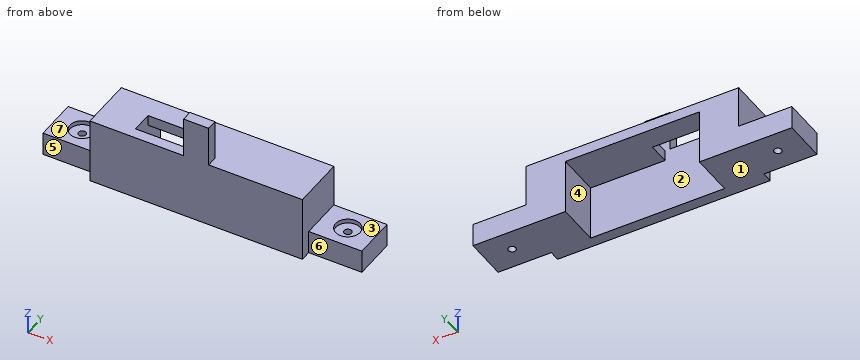
Autodesk Inventor part; units mm, degrees
ref_plane "YZ Plane" through (0, 0, 0) normal (1, 0, 0) x (0, 1, 0)
ref_plane "XZ Plane" through (0, 0, 0) normal (0, 1, 0) x (-1, 0, 0)
ref_plane "XY Plane" through (0, 0, 0) normal (0, 0, 1) x (1, 0, 0)
sketch "Sketch1" plane through (0, 0, 0) normal (0, 1, 0) x (-1, 0, 0)
  line L0 (50, -15.5) -> (-50, -15.5)
  line L1 (-50, -15.5) -> (-50, 15.5)
  line L2 (-50, 15.5) -> (50, 15.5)
  line L3 (50, 15.5) -> (50, -15.5)
  line L4 (31.5, -15.5) -> (-31.5, -15.5)
  line L5 (-31.5, -15.5) -> (-31.5, 10.5)
  line L6 (-31.5, 10.5) -> (31.5, 10.5)
  line L7 (31.5, 10.5) -> (31.5, -15.5)
  line L8 (50, -15.5) -> (75, -15.5)
  line L9 (75, -15.5) -> (75, -4.5)
  line L10 (75, -4.5) -> (50, -4.5)
  line L11 (50, -4.5) -> (50, -15.5)
  line L12 (0, 0) -> (0, -15.5)
  line L13 (-50, -15.5) -> (-75, -15.5)
  line L14 (-75, -15.5) -> (-75, -4.5)
  line L15 (-75, -4.5) -> (-50, -4.5)
  point P0 (-50, -4.5)
  point P1 (-31.5, -15.5)
  dimension "d0" = 100
  dimension "d1" = 50
  dimension "d2" = 31
  dimension "d3" = 15.5
  dimension "d4" = 26
  dimension "d5" = 63
  dimension "d6" = 31.5
  dimension "d7" = 11
  dimension "d8" = 25
extrude "Extrusion1" add sketch "Sketch1" along normal blind 20 contours L0 L7 L6 L5 L1 L2 L3 | L3 L10 L9 L8 | L13 L14 L15 L1
sketch "Sketch2" plane through (-75, 0, -4.5) normal (0, 0, 1) x (1, 0, 0)
  line L0 (0, 0) -> (25, 0)
  line L1 (25, 0) -> (25, 20)
  line L2 (0, 20) -> (25, 20)
  line L3 (0, 0) -> (0, 20)
  circle A0 centre (12.5, 10) radius 1.75
  circle A1 centre (12.5, 10) radius 5.75
  point P0 (75, 0)
  dimension "d11" = 3.5
  dimension "d12" = 11.5
extrude "Extrusion2" cut sketch "Sketch2" against normal through all contours A0
extrude "Extrusion3" cut sketch "Sketch2" against normal blind 2 contours A1
mirror "Mirror1" about plane through (0, 0, 0) normal (1, 0, 0) of "Extrusion3", "Extrusion2"
sketch "Sketch4" plane through (0, 0, 0) normal (0, -1, 0) x (1, 0, 0)
  line L0 (-31.5, -15.5) -> (-75, -15.5)
  line L1 (-31.5, 10.5) -> (-31.5, -15.5)
  line L2 (31.5, 10.5) -> (-31.5, 10.5)
  line L3 (31.5, -15.5) -> (31.5, 10.5)
  line L4 (75, -15.5) -> (31.5, -15.5)
  line L5 (75, -4.5) -> (75, -15.5)
  line L6 (50, -4.5) -> (75, -4.5)
  line L7 (50, 15.5) -> (50, -4.5)
  line L8 (-50, 15.5) -> (50, 15.5)
  line L9 (-50, -4.5) -> (-50, 15.5)
  line L10 (-75, -4.5) -> (-50, -4.5)
  line L11 (-75, -15.5) -> (-75, -4.5)
  line L12 (75, -15.5) -> (31.5, -15.5)
  line L13 (50, -15.5) -> (-50, -15.5)
  line L14 (-50, -15.5) -> (-50, 34.5)
  line L15 (-50, 34.5) -> (50, 34.5)
  line L16 (50, 34.5) -> (50, -15.5)
  point P0 (0, 0)
  dimension "d22" = 100
  dimension "d23" = 50
extrude "Extrusion5" add sketch "Sketch4" along normal blind 5 contours L0 L14 L9 L8 L7 L16 L4 L3 L2 L1 | L1 L2 L3 L13 | L14 L15 L16 L8
sketch "Sketch5" plane through (31.5, 20, 10.5) normal (0, 0, -1) x (-1, 0, 0)
  line L0 (63, -20) -> (0, -20)
  line L1 (63, -20) -> (35, -20)
  line L2 (35, -20) -> (35, -10)
  line L3 (35, -10) -> (63, -10)
  line L4 (63, -10) -> (63, -20)
  point P0 (31.5, -20)
  dimension "d26" = 28
  dimension "d27" = 10
extrude "Extrusion6" cut sketch "Sketch5" against normal blind 57
sketch "Sketch6" plane through (0, 0, 0) normal (0, 1, 0) x (1, 0, 0)
  line L0 (-50, -15.5) -> (-31.5, -15.5)
  line L1 (-50, -34.5) -> (-50, -15.5)
  line L2 (50, -34.5) -> (-50, -34.5)
  line L3 (50, -15.5) -> (50, -34.5)
  line L4 (-3.5, -15.5) -> (50, -15.5)
  line L5 (-3.5, -10.5) -> (-3.5, -15.5)
  line L6 (31.5, -10.5) -> (-3.5, -10.5)
  line L7 (31.5, 15.5) -> (31.5, -10.5)
  line L8 (-31.5, 15.5) -> (31.5, 15.5)
  line L9 (-31.5, 15.5) -> (-31.5, -15.5)
  line L10 (-0.0641, -15.5) -> (-0.0641, -32.5)
  line L11 (-0.0641, -32.5) -> (-0.0641, -22.5) construction
  line L12 (0.7628, -32.5) -> (0.7628, -22.5)
  line L13 (-0.891, -22.5) -> (-0.891, -32.5)
  arc A0 (-0.891, -32.5) -> (0.7628, -32.5) centre (-0.0641, -32.5) ccw
  arc A1 (0.7628, -22.5) -> (-0.891, -22.5) centre (-0.0641, -22.5) ccw
  point P0 (0, 0)
  point P1 (-0.0641, -27.5)
  dimension "d36" = 10
  dimension "d37" = 2
extrude "Extrusion7" cut sketch "Sketch6" against normal blind 2 contours A1 L12 A0 L13
sketch "Sketch7" plane through (0, 0, 0) normal (0, 1, 0) x (1, 0, 0)
  line L0 (-3.5, -10.5) -> (-3.5, -15.5)
  arc A0 (-0.891, -32.5) -> (0.7628, -32.5) centre (-0.0641, -32.5) ccw
  line L1 (-0.891, -32.5) -> (-0.891, -22.5)
  arc A1 (0.7628, -22.5) -> (-0.891, -22.5) centre (-0.0641, -22.5) ccw
  line L2 (0.7628, -22.5) -> (0.7628, -32.5)
  line L3 (-50, -15.5) -> (-31.5, -15.5)
  line L4 (-50, -34.5) -> (-50, -15.5)
  line L5 (50, -34.5) -> (-50, -34.5)
  line L6 (50, -15.5) -> (50, -34.5)
  line L7 (-3.5, -15.5) -> (50, -15.5)
  line L8 (-3.5, -10.5) -> (-3.5, -15.5)
  line L9 (31.5, -10.5) -> (-3.5, -10.5)
  line L10 (31.5, 15.5) -> (31.5, -10.5)
  line L11 (-31.5, 15.5) -> (31.5, 15.5)
  line L12 (-31.5, 15.5) -> (-31.5, -15.5)
  line L13 (-3.5, -15.5) -> (50, -15.5)
  line L14 (50, -34.5) -> (-50, -34.5)
  line L15 (-3.5, -15.5) -> (-50, -15.5)
  line L16 (-50, -15.5) -> (-50, -34.5)
  line L17 (-50, -34.5) -> (-3.5, -34.5)
  line L18 (-3.5, -34.5) -> (-3.5, -15.5)
  line L19 (-50, -15.5) -> (50, -15.5)
  line L20 (-5.891, -34.5) -> (-50, -34.5)
  line L21 (-50, -34.5) -> (-50, -15.5)
  line L22 (-50, -15.5) -> (-5.891, -15.5)
  line L23 (-5.891, -15.5) -> (-5.891, -34.5)
  point P0 (0, 0)
  point P1 (-5.891, -34.5)
  point P2 (-5.891, -15.5)
  dimension "d32" = 5
extrude "Extrusion8" cut sketch "Sketch7" against normal blind 24.25 contours L23 L5 L4 L3 L15
mirror "Mirror2" about plane through (0, 0, 0) normal (1, 0, 0) of "Extrusion8"
sketch "Sketch10" plane through (0, 0, 0) normal (0, 1, 0) x (1, 0, 0)
  line L0 (-3.5, -10.5) -> (-3.5, -15.5)
  arc A0 (0.7628, -22.5) -> (-0.891, -22.5) centre (-0.0641, -22.5) ccw
  line L1 (0.7628, -22.5) -> (0.7628, -32.5)
  arc A1 (-0.891, -32.5) -> (0.7628, -32.5) centre (-0.0641, -32.5) ccw
  line L2 (-0.891, -32.5) -> (-0.891, -22.5)
  line L3 (5.891, -34.5) -> (5.891, -15.5)
  line L4 (-3.5, -15.5) -> (5.891, -15.5)
  line L5 (-3.5, -10.5) -> (-3.5, -15.5)
  line L6 (31.5, -10.5) -> (-3.5, -10.5)
  line L7 (31.5, 15.5) -> (31.5, -10.5)
  line L8 (-31.5, 15.5) -> (31.5, 15.5)
  line L9 (-31.5, 15.5) -> (-31.5, -15.5)
  line L10 (-31.5, -15.5) -> (-5.891, -15.5)
  line L11 (-5.891, -15.5) -> (-5.891, -34.5)
  line L12 (5.891, -34.5) -> (-5.891, -34.5)
  line L13 (-3.5, -15.5) -> (3.4148, -15.5)
  line L14 (3.4148, -15.5) -> (3.4148, -19.7081)
  line L15 (3.4148, -19.7081) -> (-3.5, -19.7081)
  line L16 (-3.5, -19.7081) -> (-3.5, -15.5)
  point P0 (0, 0)
equation "\"d1\" = 0.5 * d0"
equation "\"d3\" = 0.5 * d2"
equation "\"d6\" = 0.5 * d5"
properties part number "blah"
Work out the finished part from the listing and answer in its coordinate system (mm). Face numbers are marked on the shaded views. A direction names the side the tool comes from. Give positions to 0.01 mm unless a question says otherwise; leave off trailing zeros. Loops run counter-clockwise (first coordinate to the right, second up) from the corner with the lowest first, then second, coordinate; pieces in that order, holes last. Notation, with made-up numbers: (13, 64.25) - (30, 64.25) arc R22 ccw to (30, 81.25) - close; hole circle Ø1 at (-23, 17). An arc over 180 degrees is marked (long way). Answer in a Markdown table with one row per item.
(1) A tool of negligible diameter and unlimited length cuts with its end or side. For the marked faces 3, 4, 5, 6 and 7, from which of +Z, -Z, +X, -X, +Y, -Y can it reach the whole face along a straight path? Write none if from no direction.
Results list:
| item | result |
|---|---|
| face 3 | +Z, +X, +Y, -Y |
| face 4 | -Z, +Y |
| face 5 | +Z, -Z, -X, -Y |
| face 6 | +Z, -Z, +X, -Y |
| face 7 | +Z, -X, +Y, -Y |
(2) Section C-C (z = -10) is taken. Give the vertices of the cut face in (x, y), and give its area (3 significant figures).
Results list:
| item | result |
|---|---|
| outline | (-75, 0) - (-50, 0) - (-50, -5) - (50, -5) - (50, 0) - (75, 0) - (75, 20) - (31.5, 20) - (31.5, 0) - (-31.5, 0) - (-31.5, 20) - (-75, 20) - close; hole circle Ø3.5 at (-62.5, 10); hole circle Ø3.5 at (62.5, 10) |
| area | 2,220 mm² |
(3) Consider L1, parallel to X at y = 9.5, z = -5.5; L2, parallel to X at y = 6.25, z = 14.5; L3, parallel to X at y = 7.75, z = 10. Determine where each line is inside the solid, lowest interval first. Write a range as [from, to].
Results list:
| item | result |
|---|---|
| L1 | x = [-75, -68.23], [-56.77, -31.5], [31.5, 56.77], [68.23, 75] |
| L2 | x = [-50, -31.5], [-3.5, 50] |
| L3 | x = [-50, -31.5], [31.5, 50] |
(4) Section D-D (z = -1) is taken. Give the vertices of the cut face in (x, y).
Results list:
| item | result |
|---|---|
| outline | (-50, -5) - (50, -5) - (50, 20) - (31.5, 20) - (31.5, 0) - (-31.5, 0) - (-31.5, 20) - (-50, 20) - close |
(5) For a pull along X with two mould halves and no side action, classify the marked faces 1 and 2 as pulls with the +X half, pulls with the -X half, needs draft (parallel to the pull), parting line crosses it, or undercut.
Results list:
| item | result |
|---|---|
| face 1 | needs draft |
| face 2 | undercut |
(6) Section A-A (x = 62.5) is taken. Give the vertices of the cut face in (y, z).
Results list:
| item | result |
|---|---|
| outline | (0, -15.5) - (8.25, -15.5) - (8.25, -6.5) - (4.25, -6.5) - (4.25, -4.5) - (0, -4.5) - close; (11.75, -15.5) - (20, -15.5) - (20, -4.5) - (15.75, -4.5) - (15.75, -6.5) - (11.75, -6.5) - close |
(7) Section B-B (y = 2) is taken. Give the vertices of the cut face in (x, z), and give its area (3 significant figures).
Results list:
| item | result |
|---|---|
| outline | (-75, -15.5) - (-31.5, -15.5) - (-31.5, 15.5) - (-50, 15.5) - (-50, -4.5) - (-75, -4.5) - close; (-3.5, 10.5) - (31.5, 10.5) - (31.5, -15.5) - (75, -15.5) - (75, -4.5) - (50, -4.5) - (50, 15.5) - (-3.5, 15.5) - close |
| area | 1,870 mm² |
(8) Flat-ended cylindrical pins translate along their axes: pin 1 Ø6 at (x, z) = (30, -3.5) entering from +Y; pin 2 Ø1.5 at (y, z) = (-1.5, 26.5) entering from -X; pin 3 Ø1.5 at (y, z) = (-3.5, 28.5) entering from +X; pin 4 Ø10 at (x, y) = (-20.5, 9) entering from +Z. Find the tip coordinate at first contact, or state that the pin passes through.
Results list:
| item | result |
|---|---|
| pin 1 | stops at y = 20 |
| pin 2 | stops at x = -5.89 |
| pin 3 | stops at x = 5.89 |
| pin 4 | stops at z = 15.5 |
